Build history of the part. All positions in model axes, mm. Face numbers are marked on the shaded views. A direction names the side the tool comes from. Coordinates: 2 decimals unless noted, no trailing zeros. Loops run counter-clockwise (first coordinate to the right, second up) from the corner with the lowest first, then second, coordinate; pieces in that order, holes last. Notation, with made-up numbers: (17, -30.75) - (27, -30.75) arc R18 cw to (27, -6.75) - close; hole circle Ø6 at (19, -8). An arc over 180 degrees is marked (long way). One line per item, written item: value.
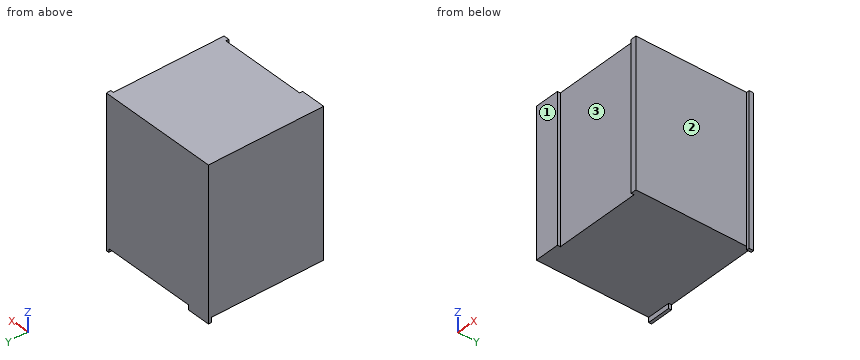
```python
from build123d import *

# Parameters (mm, degrees)
SKETCH1_W           = 1200
SKETCH1_H           = 1150
BOSS_EXTRUDE1_DEPTH = 1500
SKETCH2_W           = 57.803468208
SKETCH2_H           = 1500
SKETCH2_W_2         = 253.585640565
BOSS_EXTRUDE2_DEPTH = 30
SKETCH3_W           = 1536.946487479
SKETCH3_H           = 47.081819152
BOSS_EXTRUDE3_DEPTH = 30
SKETCH4_W           = 239.993344336
SKETCH4_H           = 1550
BOSS_EXTRUDE5_DEPTH = 30


with BuildPart() as part:
    # Sketch1 → Boss-Extrude1 (new body)
    with BuildSketch(Plane.XY):
        with Locations((-542.196531792, -155.924855491)):
            Rectangle(SKETCH1_W, SKETCH1_H)
    extrude(amount=BOSS_EXTRUDE1_DEPTH)

    # Sketch2 → Boss-Extrude2 (add)
    with BuildSketch(Plane.XZ.offset(730.924855491)):
        with Locations((28.901734104, 750)):
            Rectangle(SKETCH2_W, SKETCH2_H)
        with Locations((-1015.403711509, 750)):
            Rectangle(SKETCH2_W_2, SKETCH2_H)
    extrude(amount=BOSS_EXTRUDE2_DEPTH)

    # Sketch3 → Boss-Extrude3 (add)
    with BuildSketch(Plane(origin=(57.803468208, 0, 0), x_dir=(0, 0, -1), z_dir=(1, 0, 0))):
        with Locations((-731.52675626, 395.534234933)):
            Rectangle(SKETCH3_W, SKETCH3_H)
    extrude(amount=BOSS_EXTRUDE3_DEPTH)

    # Sketch4 → Boss-Extrude5 (add)
    with BuildSketch(Plane(origin=(0, 419.075144509, 0), x_dir=(1, 0, 0), z_dir=(0, 1, 0))):
        with Locations((-1022.199859624, -725)):
            Rectangle(SKETCH4_W, SKETCH4_H)
    extrude(amount=-BOSS_EXTRUDE5_DEPTH)


solid = part.part
```
Item 1: Cut at D-D, the plane x = -965.5. Write the cut outline in (y, z), then the cut area to 3 significant figures.
Check result:
outline: (-760.92, 0) - (389.08, 0) - (389.08, -50) - (419.08, -50) - (419.08, 1500) - (-760.92, 1500) - close
area: 1,770,000 mm^2
Item 2: Tool access for the marked faces 1, 2 and 3: list every direction of +Z, -Z, +X, -X, +Y, -Y with a clear straight run to the whole face (end or side of a thin tool).
Check result:
face 1: +Z, -Z, +X, -X, -Y
face 2: +Z, -Z, +X, -Y
face 3: +Z, -Z, -Y
Item 3: Probe probe 1 along Z at (x, y) = (-1046, -9.5); probe 2 along Y at (x, z) = (-862, 320.5); probe 3 along X at (y, z) = (-116, 1258). List the from-to ranges inside material, lowest first. Write a range as from..to.
Check result:
probe 1: z = 0..1500
probe 2: y = -730.92..419.08
probe 3: x = -1142.2..57.8
Item 4: Drop flat-ended pins along their axis: P1, Ø2, axis at x = -606.5, z = 711, coming from the -Y side; P2, Ø9, axis at x = 71, y = 389.5, coming from the -Z side; P3, Ø15, axis at x = 70, z = 805.5, coming from the -Y side. Give the stop position or say it passes through.
Check result:
P1: stops at y = -730.92
P2: stops at z = -36.95
P3: stops at y = 371.99
Item 5: Cut at C-C, the plane x = -532.5. Write the cut outline in (y, z).
Check result:
outline: (-730.92, 0) - (419.08, 0) - (419.08, 1500) - (-730.92, 1500) - close
Item 6: Cut at B-B, the plane y = 14. Write the cut outline in (x, z).
Check result:
outline: (-1142.2, 0) - (57.8, 0) - (57.8, 1500) - (-1142.2, 1500) - close
Item 7: Cut at A-A, the plane z = 231. Write the cut outline in (x, y).
Check result:
outline: (-1142.2, -760.92) - (-888.61, -760.92) - (-888.61, -730.92) - (0, -730.92) - (0, -760.92) - (57.8, -760.92) - (57.8, 371.99) - (87.8, 371.99) - (87.8, 419.08) - (-1142.2, 419.08) - close
